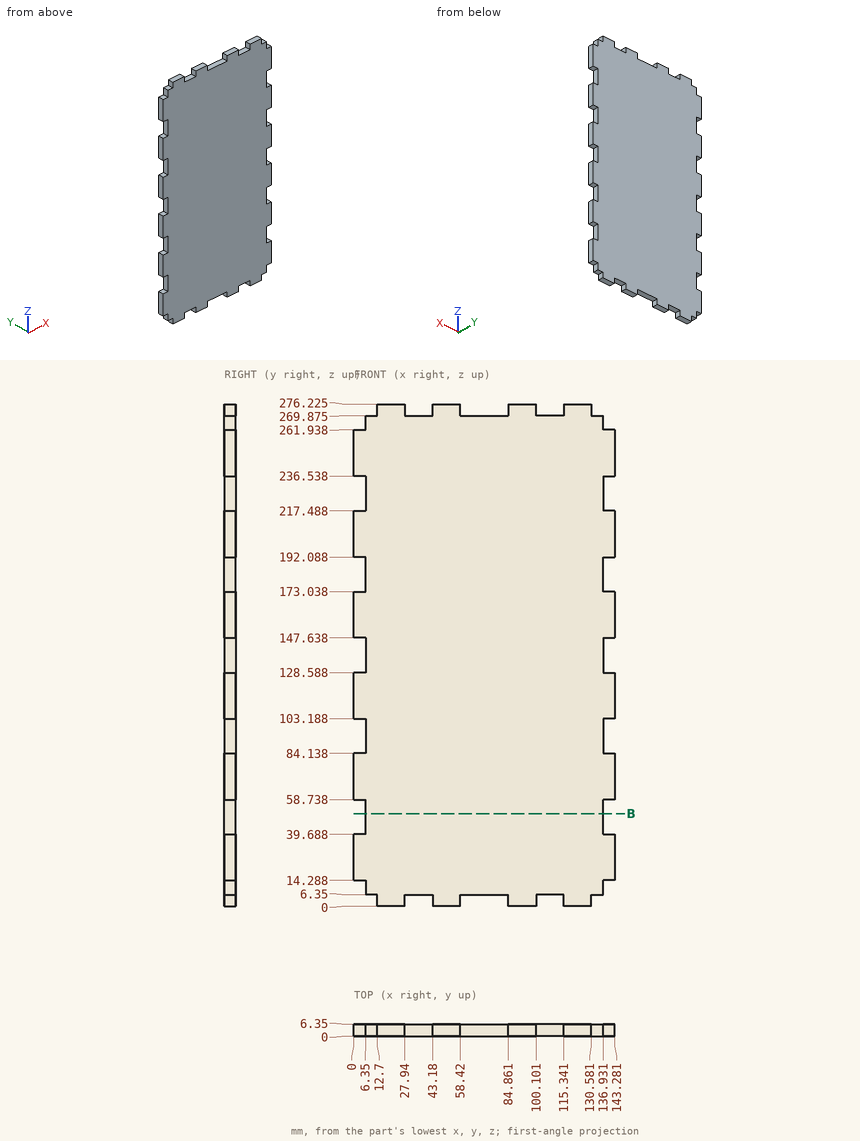
Study the drawing (mm; zero at the part's minimum x, y, z) and answer. Coordinates: 2 decimals unless noted, no trailing zeros. Loops run counter-clockwise (first coordinate to the right, second up) from the corner with the lowest first, then second, coordinate; pieces in that order, holes last. Notation, with made-up numbers: M -25.5,60 L -0.5,60 A15 cw -0.5,65 Z; hole C 68.5,40 d8. An arc over 180 degrees is marked long. Answer as a JSON object with one key per item and string values. Group by question number.
Item 1: Each of these flat-tipped pins is pushed along its axis until it touches: P1, Ø1.9, axis at x = 39, y = 4, coming from the -Z side; P2, Ø1.5, axis at x = 126, z = 38.5, coming from the -Y side; P3, Ø3, axis at x = 4.5, y = 2, coming from the -Z side; P4, Ø1.9, axis at y = 2.5, z = 3.5, coming from the +X side. Where does it stop, or does it pass through?
Item 2: Section B-B (z = 51) is taken. Write down the section's boundary in (x, y).
Item 3: Consider L1, parallel to Z at x = 137.5, y = 2.5; L2, parallel to X at y = 5, z = 176. Determine where each line is inside the solid, lowest interval first.
Solved:
{
 "1": {"P1": "stops at z = 6.35", "P2": "stops at y = 0", "P3": "stops at z = 14.29", "P4": "stops at x = 130.58"},
 "2": {"outline": "M 6.35,0 L 136.93,0 L 136.93,6.35 L 6.35,6.35 Z"},
 "3": {"L1": "z = 14.29 to 39.69, 58.74 to 84.14, 103.19 to 128.59, 147.64 to 173.04, 192.09 to 217.49, 236.54 to 261.94", "L2": "x = 6.35 to 136.93"}
}
